Geometry: final body of the model. Coordinates: model frame, mm. Coordinates: 2 decimals unless noted, no trailing zeros. Order: outer loops, then holes, each group sorted by start corner. A loop starts at its lowest first (then second) coordinate and runs counter-clockwise, first axis right, second up. Notation, with made-up numbers: M 42,5.5 L 95,5.5 A37 cw 95,44.5 Z; hole C 24.5,83.25 d3. An arc over 180 degrees is marked long. Use CSV: the item, a comma, the result in double quotes. Start each with the question number.
Q1. Section query B-B, the plane z = 0.1. Output: boundary loops of the cut face in (x, y).
Q2. Section query D-D, the plane y = -4. Output: boundary loops of the cut face in (x, z).
Q3. Ray query, probe 1 along X at (y, z) = (-3.25, 0.15); probe 2 along X at (y, z) = (-6, 0.25); probe 3 along Y at (x, z) = (19, 0.2). Return the intervals inside material, ascending.
Q4. Section query A-A, the plane y = 4.75. Output: boundary loops of the cut face in (x, z).
Q5. Section query C-C, the plane x = 60.95. Output: boundary loops of the cut face in (y, z).
from build123d import *

# Parameters (mm, degrees)
F1_DEPTH = 0.3


with BuildPart() as f1:
    # F0 (on Top) → F1 (new body)
    with BuildSketch(Plane.XY):
        with BuildLine():
            ThreePointArc((53, -8.25), (60.95, -0.3), (68.9, -8.25))
            Line((68.9, -8.25), (102.9, -8.25))
            Line((102.9, -8.25), (102.9, 8.25))
            Line((102.9, 8.25), (87.9, 8.25))
            ThreePointArc((87.9, 8.25), (79.95, 0.3), (72, 8.25))
            Line((72, 8.25), (49.9, 8.25))
            ThreePointArc((49.9, 8.25), (41.95, 0.3), (34, 8.25))
            Line((34, 8.25), (0, 8.25))
            Line((0, 8.25), (0, -8.25))
            Line((0, -8.25), (15, -8.25))
            ThreePointArc((15, -8.25), (22.95, -0.3), (30.9, -8.25))
            Line((30.9, -8.25), (53, -8.25))
        make_face()
    extrude(amount=F1_DEPTH)


solid = f1.part
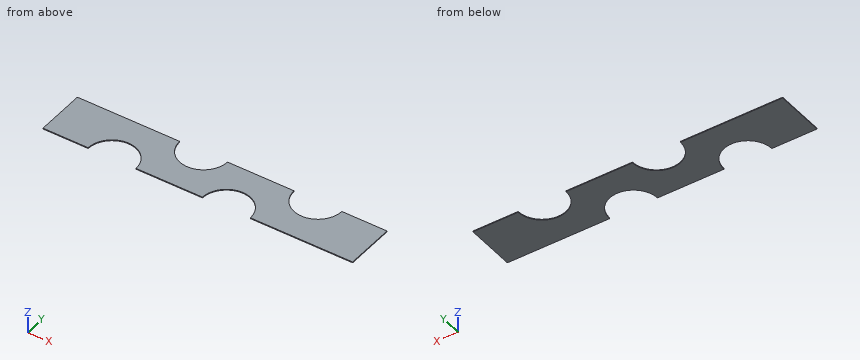
Responses:
1,outline,"M 0,-8.25 L 15,-8.25 A7.95 cw 30.9,-8.25 L 53,-8.25 A7.95 cw 68.9,-8.25 L 102.9,-8.25 L 102.9,8.25 L 87.9,8.25 A7.95 cw 72,8.25 L 49.9,8.25 A7.95 cw 34,8.25 L 0,8.25 Z"
2,outline,"M 0,0 L 16.23,0 L 16.23,0.3 L 0,0.3 Z; M 29.67,0 L 54.23,0 L 54.23,0.3 L 29.67,0.3 Z; M 67.67,0 L 102.9,0 L 102.9,0.3 L 67.67,0.3 Z"
3,probe 1,"x = 0 to 16.77, 29.13 to 54.77, 67.13 to 102.9"
3,probe 2,"x = 0 to 15.33, 30.57 to 53.33, 68.57 to 102.9"
3,probe 3,"y = -1.35 to 8.25"
4,outline,"M 0,0 L 34.81,0 L 34.81,0.3 L 0,0.3 Z; M 49.09,0 L 72.81,0 L 72.81,0.3 L 49.09,0.3 Z; M 87.09,0 L 102.9,0 L 102.9,0.3 L 87.09,0.3 Z"
5,outline,"M -0.3,0 L 8.25,0 L 8.25,0.3 L -0.3,0.3 Z"
